from build123d import *
from build123d.topology import SkipClean

# Parameters (mm, degrees)
STOCK_GOUX_START         = 53.391336338
STOCK_GOUX_LIKED_1_DEPTH = 20.568134432
CUT_EXTRUDE1_DEPTH       = 109.511360444
BOSS_EXTRUDE1_DEPTH      = 20.568134
FILLET1_R                = 12.7
SKETCH3_R                = 0.64999997
CUT_EXTRUDE2_DEPTH       = 149.612005727
CUT_EXTRUDE3_DEPTH       = 0.4


# Read off the part's stored shape, not the designer's step: Stock-Goux Liked-1
with BuildPart() as part:
    # Stock-Goux Liked-1 outline → Stock-Goux Liked-1 (new body)
    with BuildSketch(Plane(origin=(0, 0, 0), x_dir=(0.8164965809277512, -0.4082482904637994, -0.40824829046387656), z_dir=(0.5773502691895902, 0.5773502691895891, 0.5773502691896982)).offset(STOCK_GOUX_START)):
        Polygon((57.433440297, -119.932119095), (57.866453013, -120.182119103), (60.366452966, -115.851992166), (63.397541976, -117.601992222), (65.647541921, -113.704878), (70.147541811, -113.704878), (70.147541811, -110.204877888), (75.147541717, -110.204877888), (75.147541717, -109.704877872), (63.338140771, -109.704877872), align=None)
    extrude(amount=STOCK_GOUX_LIKED_1_DEPTH)

    # Sketch1 → Cut-Extrude1 (cut, through all)
    with BuildSketch(Plane(origin=(0, -80.401490288, 80.401490288), x_dir=(1, 0, 0), z_dir=(0, -0.7071067811865477, 0.7071067811865475))):
        Polygon((84.426495932, 5.692217571), (86.735897009, 8.958203895), (94.492614361, 3.473376455), (92.183213285, 0.207390132), align=None)
        Polygon((96.301513883, 22.486029011), (104.058231236, 17.001201571), (101.748830159, 13.735215248), (93.992112807, 19.220042687), align=None)
    extrude(amount=-CUT_EXTRUDE1_DEPTH, mode=Mode.SUBTRACT)

    # Sketch2 → Boss-Extrude1 (add)
    with SkipClean():  # the faces are left unmerged after this step: merging them gives an invalid solid
        with BuildSketch(Plane(origin=(30.825502407, 30.825502407, 30.825502407), x_dir=(-0.40824829046391425, -0.4082482904639143, 0.8164965809276746), z_dir=(-0.5773502691895895, -0.5773502691895894, -0.5773502691896983))):
            Polygon((62.183440195, -111.704877936), (65.647541921, -113.704878), (67.897541921, -109.807763683), (64.433440195, -107.807763619), align=None)
        extrude(amount=-BOSS_EXTRUDE1_DEPTH)

    # Fillet1
    fillet1_edges = [part.edges().sort_by_distance(p)[0] for p in [
        (86.689770169, -68.456355976, 92.055619581),
    ]]
    fillet(fillet1_edges, radius=FILLET1_R)

    # Sketch3 → Cut-Extrude2 (cut, through all)
    with SkipClean():  # the faces are left unmerged after this step: merging them gives an invalid solid
        with BuildSketch(Plane(origin=(53.600993525, -26.800496763, -26.800496763), x_dir=(-0.36514837167009556, 0.18257418583503127, -0.9128709291752878), z_dir=(0.8164965809277506, -0.40824829046383865, -0.4082482904638387))):
            with Locations(Location((-132.231040931, -15.066915515, 0), (0, 0, 348.463040967))):
                Circle(SKETCH3_R)
        cut_extrude2 = extrude(amount=-CUT_EXTRUDE2_DEPTH, mode=Mode.SUBTRACT)

    # Mirror1: Cut-Extrude2 across plane
    with SkipClean():  # the faces are left unmerged after this step: merging them gives an invalid solid
        add(cut_extrude2.mirror(Plane(origin=(36.763011383, 36.763011383, 36.763011383), x_dir=(-0.40824829046390154, -0.40824829046390165, 0.8164965809276874), z_dir=(0.5773502691895985, 0.5773502691895986, 0.5773502691896802))), mode=Mode.SUBTRACT)

    # Sketch4 → Cut-Extrude3 (cut)
    with SkipClean():  # the faces are left unmerged after this step: merging them gives an invalid solid
        with BuildSketch(Plane(origin=(0, -77.573063073, 77.573063073), x_dir=(1, 0, 0), z_dir=(0, 0.7071067811865477, -0.7071067811865475))):
            with BuildLine():
                Line((93.057379032, -13.173091082), (92.567645459, -13.519084672))
                Line((92.567645459, -13.519084672), (91.270169497, -11.686081867))
                Line((91.270169497, -11.686081867), (89.687757638, -12.423862316))
                add(Edge.make_bspline(
                    [(89.687757638, -12.423862316), (89.741295568, -12.46776154), (89.844942898, -12.552748714), (89.986729771, -12.686351444), (90.109493379, -12.820951582), (90.180253462, -12.914346072), (90.214380234, -12.959389159)],
                    knots=[0, 0, 0, 0, 1.102510947, 2.134417912, 3.100251258, 4, 4, 4, 4], degree=3))
                add(Edge.make_bspline(
                    [(90.214380234, -12.959389159), (90.253760272, -13.017586925), (90.331220007, -13.132060751), (90.424525722, -13.313424806), (90.499954525, -13.496549573), (90.552853451, -13.683170388), (90.588524358, -13.872165751), (90.600192512, -14.064230957), (90.594316704, -14.258572886), (90.567052813, -14.453627198), (90.522232401, -14.646119682), (90.456443819, -14.831644428), (90.37370764, -15.009053992), (90.272718514, -15.178186861), (90.151902914, -15.337992616), (90.012792553, -15.489286627), (89.855636039, -15.632722917), (89.740254809, -15.718962844), (89.681397462, -15.762954864)],
                    knots=[0, 0, 0, 0, 1.053566777, 2.072344485, 3.054154547, 4.020735706, 4.977911009, 5.934388254, 6.901994919, 7.890871114, 8.884708514, 9.862655974, 10.838946315, 11.817700602, 12.812779523, 13.839512687, 14.897909552, 16, 16, 16, 16], degree=3))
                add(Edge.make_bspline(
                    [(89.681397462, -15.762954864), (89.638861949, -15.79180454), (89.554795968, -15.84882222), (89.424554492, -15.926036449), (89.290895408, -15.991410287), (89.155300895, -16.049553503), (89.016642135, -16.097655089), (88.875174038, -16.137099385), (88.731270115, -16.168140221), (88.585356233, -16.187761829), (88.439700765, -16.199777545), (88.296040345, -16.200730613), (88.155005398, -16.193081949), (88.016337233, -16.176925914), (87.879820972, -16.150143257), (87.746101629, -16.112905095), (87.614836668, -16.066952156), (87.486042986, -16.012633338), (87.36135061, -15.94736132), (87.240735277, -15.873163467), (87.122735013, -15.792270246), (87.011070103, -15.699661066), (86.902568847, -15.599581488), (86.800066565, -15.489353904), (86.699506263, -15.37226378), (86.638126187, -15.288079908), (86.606888247, -15.245236515)],
                    knots=[0, 0, 0, 0, 1.059045057, 2.093066608, 3.116885153, 4.123102215, 5.131744447, 6.138757912, 7.148156815, 8.162686115, 9.170608983, 10.158022319, 11.120612269, 12.079785529, 13.032569554, 13.984391495, 14.937776329, 15.896949589, 16.862272095, 17.834843879, 18.814104655, 19.80760772, 20.82157244, 21.85385735, 22.907771379, 24, 24, 24, 24], degree=3))
                add(Edge.make_bspline(
                    [(86.606888247, -15.245236515), (86.571580982, -15.193252636), (86.502142451, -15.091016336), (86.41618388, -14.93004522), (86.344744771, -14.767482877), (86.292163209, -14.601805216), (86.252344887, -14.434043372), (86.233224181, -14.263324381), (86.227400474, -14.090507286), (86.239494355, -13.916834049), (86.265515908, -13.744722824), (86.30797018, -13.577552607), (86.364080119, -13.416020283), (86.435375705, -13.260390942), (86.522836864, -13.111119621), (86.623492387, -12.96724671), (86.738046259, -12.828566566), (86.824857153, -12.744064342), (86.86892751, -12.701166002)],
                    knots=[0, 0, 0, 0, 1.073683973, 2.111606131, 3.114875596, 4.105229039, 5.079452871, 6.057740752, 7.036807216, 8.032083212, 9.029653356, 10.008961322, 10.976446223, 11.949563641, 12.930560464, 13.930051518, 14.949171403, 16, 16, 16, 16], degree=3))
                Line((86.86892751, -12.701166002), (87.244177911, -13.230332668))
                add(Edge.make_bspline(
                    [(87.244177911, -13.230332668), (87.203630602, -13.274365386), (87.125511073, -13.359199998), (87.030245223, -13.496920616), (86.953711988, -13.633102202), (86.89891325, -13.771272529), (86.866072042, -13.912811297), (86.849115424, -14.058372065), (86.851210509, -14.209486442), (86.86900954, -14.363314897), (86.902300542, -14.516992644), (86.955818974, -14.664132133), (87.020988019, -14.806766078), (87.078858378, -14.893581403), (87.108070138, -14.937403982)],
                    knots=[0, 0, 0, 0, 1.151825873, 2.219138558, 3.21719232, 4.156104017, 5.071411429, 6.008616142, 6.972493179, 7.975548077, 8.988201805, 9.993150609, 10.986983969, 12, 12, 12, 12], degree=3))
                add(Edge.make_bspline(
                    [(87.108070138, -14.937403982), (87.138555874, -14.978424636), (87.19858351, -15.059195946), (87.303110462, -15.166361235), (87.415414903, -15.261227558), (87.537005465, -15.343065931), (87.667525961, -15.411983911), (87.80637932, -15.468149642), (87.954429953, -15.510207129), (88.109024438, -15.538668693), (88.267373598, -15.554853821), (88.425830222, -15.552517547), (88.58235856, -15.538339817), (88.736728883, -15.505941209), (88.888199475, -15.456572805), (89.039090754, -15.394670176), (89.187152138, -15.315407609), (89.281232645, -15.252012671), (89.329043696, -15.219795809)],
                    knots=[0, 0, 0, 0, 0.982901861, 1.935373165, 2.873857243, 3.808820726, 4.750847603, 5.710288131, 6.686831843, 7.708192972, 8.733167937, 9.745322852, 10.754049183, 11.754552243, 12.77418333, 13.817071584, 14.890651141, 16, 16, 16, 16], degree=3))
                add(Edge.make_bspline(
                    [(89.329043696, -15.219795809), (89.37068488, -15.188638571), (89.452236147, -15.127619358), (89.563587258, -15.026915322), (89.660802629, -14.919270083), (89.74548165, -14.805974644), (89.815581792, -14.685946996), (89.872085801, -14.560060608), (89.915042433, -14.428675913), (89.946372379, -14.292531636), (89.960656297, -14.1529597), (89.963134707, -14.01262796), (89.946603574, -13.872900372), (89.917624638, -13.733424144), (89.872568669, -13.594113504), (89.812188994, -13.455718618), (89.738492589, -13.316631534), (89.678065145, -13.22849889), (89.64705251, -13.183267364)],
                    knots=[0, 0, 0, 0, 1.074728317, 2.104778202, 3.097685251, 4.068882731, 5.023484141, 5.965079531, 6.915809939, 7.876988247, 8.846879582, 9.811090509, 10.772268818, 11.748712747, 12.75216451, 13.792604211, 14.867118046, 16, 16, 16, 16], degree=3))
                add(Edge.make_bspline(
                    [(89.64705251, -13.183267364), (89.618173393, -13.145235048), (89.558752843, -13.066981231), (89.459652489, -12.952007275), (89.34552654, -12.839732315), (89.220663354, -12.725514625), (89.081587528, -12.612997782), (88.930468675, -12.499599482), (88.765496982, -12.387822996), (88.650403504, -12.314998695), (88.591263247, -12.277578261)],
                    knots=[0, 0, 0, 0, 0.818651868, 1.684426275, 2.599403717, 3.561756698, 4.584719662, 5.664970434, 6.800155744, 8, 8, 8, 8], degree=3))
                Line((88.591263247, -12.277578261), (91.48132735, -10.945757348))
                Line((91.48132735, -10.945757348), (93.057379032, -13.173091082))
            make_face()
        extrude(amount=-CUT_EXTRUDE3_DEPTH, mode=Mode.SUBTRACT)


solid = part.part
Model file for the job. Use its own axes, mm. A direction names the side the tool comes from. Give positions to 0.01 mm unless a question says otherwise; leave off trailing zeros. Loops run counter-clockwise (first coordinate to the right, second up) from the corner with the lowest first, then second, coordinate; pieces in that order, holes last. Notation, with made-up numbers: (21, -4) - (36, -4) arc R13 ccw to (36, 10) - close; hole circle Ø3 at (15, 6.25). An arc over 180 degrees is marked (long way). Use one line per item in the form item = value.
(1) Drop flat-ended pins along their axis: P1, Ø10, axis at y = -69, z = 90, coming from the -X side; P2, Ø3, axis at x = 82, y = -74, coming from the -Z side; P3, Ø1.5, axis at x = 96.5, z = 84.5, coming from the +Y side; P4, Ø1, axis at x = 81.5, y = -67.5, coming from the +Z side. Give the stop position or say it passes through.
Determined:
P1 = 81.12
P2 = 82.36
P3 = -69.9
P4 = through
(2) Drill centre lines: L1, parallel to X at y = -74, z = 85; L2, parallel to Z at x = 99.75, y = -67.5; L3, parallel to X at y = -63.75, z = 95. Where is each one in solid material? Low to high.
Determined:
L1 = 81.48 to 84.17, 85.71 to 85.9, 88.4 to 91.41
L2 = 87.65 to 88.35
L3 = 90.29 to 92.39, 94.39 to 96.03
(3) Pull direction Z, two halves, no side cores. Call faces 1 (the face through (96.2, -66.52, 91.49)), 2 (the face through (83.368, -73.604, 85.274)), 3 (the face through (86.607, -65.997, 89.43)), 4 (the face through (90.49, -69.19, 86.23)): pulls with the +Z half, pulls with the -Z half, needs draft (parallel to the pull), parting line crosses it, or undercut.
Determined:
face_1 = undercut
face_2 = undercut
face_3 = pulls with the +Z half
face_4 = pulls with the -Z half
(4) Cut at A-A (x = 98.5). Give the cut face in (y, z), then the cut area to 3 significant figures.
Determined:
outline = (-71.46, 84.39) - (-71.11, 84.04) - (-66.24, 88.91) - (-66.59, 89.26) - close
area = 3.45 mm^2
(5) 3-axis set-ups, long thin cutter, end or side, ignore diameter. For faces 5 (the face through (84.407, -70.739, 96.371)), 6 (the face through (85.3, -73.8, 83.6)), 7 (the face through (87.19, -71.1, 93.96)), 8 (the face through (91.928, -68.792, 86.633)), 9 (the face through (94.874, -64.22, 93.165)): which of +Z, -Z, +X, -X, +Y, -Y reach the whole face in a straight line?
Determined:
face_5 = +Z, -X, +Y
face_6 = -Z, -Y
face_7 = +Z, -Y
face_8 = -Z
face_9 = +X
